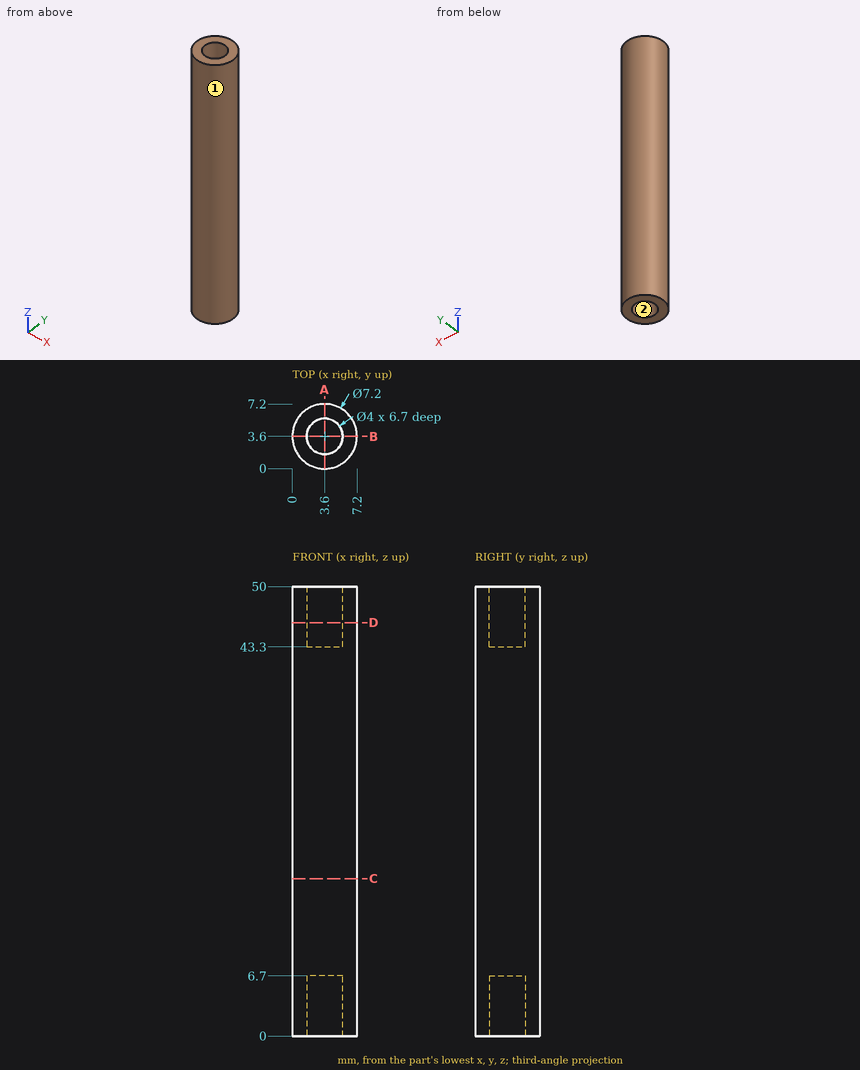
Geometry: see drawing. Coordinates: mm, zero at the bounding-box minimum. Coordinates: 2 decimals unless noted, no trailing zeros. Order: outer loops, then holes, each group sorted by start corner. A loop starts at its lowest first (then second) coordinate and runs counter-clockwise, first axis right, second up. Notation, with made-up numbers: M 31,-19 L 83,-19 A30 cw 83,15 Z; hole C 83,77 d5. An arc over 180 degrees is marked long. Write item = value, one per line. Start each with the question number.
(1) Pull-direction query (Y, two-part tool) for the marked faces 1 and 2; classes: released by +Y, released by -Y, zero draft, split by the parting line, or undercut.
(2) Section C-C on z = 17.5. Output: boundary loops of the cut face in (x, y), and give its area (3 significant figures).
(3) Line query: line 1 along Y through (x, z) = (3.6, 1.75); line 2 along Z through (x, y) = (2, 3.5); line 3 along Y through (x, z) = (3.5, 36.5). Output: solid intervals per line, ascending. Write a range as [from, to].
(4) First-contact query: P1, Ø1.5, axis at y = 1, z = 25, coming from the -X side; P2, Ø1.2, axis at x = 3, y = 4, coming from the +Z side; P3, Ø1.2, axis at x = 3, y = 2.5, coming from the -Z side. Flat tips, straight axial feed; report the tip coordinate or a pass-through.
(5) Section D-D on z = 46. Output: boundary loops of the cut face in (x, y), and give its area (3 significant figures).
(6) Section A-A on x = 3.6. Output: boundary loops of the cut face in (y, z).
Result set:
q1.face_1 = split by the parting line
q1.face_2 = undercut
q2.outline = C 3.6,3.6 d7.2
q2.area = 40.7 mm²
q3.line_1 = [0, 1.6], [5.6, 7.2]
q3.line_2 = [6.7, 43.3]
q3.line_3 = [0, 7.2]
q4.P1 = 0.51
q4.P2 = 43.3
q4.P3 = 6.7
q5.outline = C 3.6,3.6 d7.2; hole C 3.6,3.6 d4
q5.area = 28.1 mm²
q6.outline = M 0,0 L 1.6,0 L 1.6,6.7 L 5.6,6.7 L 5.6,0 L 7.2,0 L 7.2,50 L 5.6,50 L 5.6,43.3 L 1.6,43.3 L 1.6,50 L 0,50 Z
